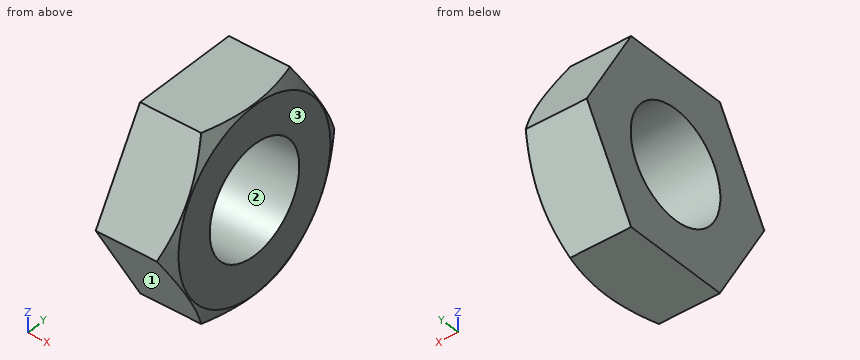
```python
from build123d import *

# Parameters (mm, degrees)
BOSS_EXTRUDE1_DEPTH        = 9
M16X2_0_TAPPED_HOLE1_D     = 14
M16X2_0_TAPPED_HOLE1_DEPTH = 9


with BuildPart() as part:
    # Sketch1 → Boss-Extrude1 (new body)
    with BuildSketch(Plane(origin=(0, 0, 0), x_dir=(0, 0, -1), z_dir=(1, 0, 0))):
        Polygon((12, 6.92820323), (0, 13.856406461), (-12, 6.92820323), (-12, -6.92820323), (0, -13.856406461), (12, -6.92820323), align=None)
    extrude(amount=-BOSS_EXTRUDE1_DEPTH)

    # M16x2.0 Tapped Hole1
    with Locations(Plane(origin=(0, 0, 0), x_dir=(0, 0, -1), z_dir=(1, 0, 0))):
        with Locations((0, 0)):
            Hole(M16X2_0_TAPPED_HOLE1_D / 2, depth=M16X2_0_TAPPED_HOLE1_DEPTH)

    # Sketch10 → Cut-Revolve1 (revolve, cut)
    with BuildSketch(Plane.XY):
        Polygon((0, 13.856406461), (0, 11.856406461), (-1.154700538, 13.856406461), align=None)
    revolve(axis=Axis((0, 0, 0), (1, 0, 0)), mode=Mode.SUBTRACT)


solid = part.part
```
Verification items for the finished model (mm, model axes). Face numbers are marked on the shaded views. Give positions to 0.01 mm unless a question says otherwise; leave off trailing zeros. Order: outer loops, then holes, each group sorted by start corner. A loop starts at its lowest first (then second) coordinate and runs counter-clockwise, first axis right, second up. Notation, with made-up numbers: (23.25, 74.5) -> (57.25, 74.5) arc R22 cw to (57.25, 102.5) -> close; hole circle Ø11 at (28, -5). An arc over 180 degrees is marked (long way). One line per item, written item: value.
(1) Draft check along Y on the marked faces 1, 2 and 3. Enter one of: pulls with the +Y half, pulls with the -Y half, needs draft (parallel to the pull), parting line crosses it, or undercut.
Final values:
face 1: pulls with the -Y half
face 2: undercut
face 3: needs draft
(2) Sectioned sample at A-A on x = -3.25. Record the cut outline in (y, z), then the cut area to 3 significant figures.
Final values:
outline: (-13.86, 0) -> (-6.93, -12) -> (6.93, -12) -> (13.86, 0) -> (6.93, 12) -> (-6.93, 12) -> close; hole circle Ø14 at (0, 0)
area: 345 mm^2
(3) Gauge pin test, flat ends, axial feed: pin 1 (1.5 mm diameter, centred on x = -7.5, y = 9, fed in from +Z); pin 2 (3 mm diameter, centred on x = -4.5, z = -9.5, fed in from +Y). Record the tip position at first contact, or that the pin passes through.
Final values:
pin 1: z = 9.71
pin 2: y = 9.24
(4) Sectioned sample at B-B on y = 0. Record the cut outline in (x, z), then the cut area to 3 significant figures.
Final values:
outline: (-9, -12) -> (-0.08, -12) -> (0, -11.86) -> (0, -7) -> (-9, -7) -> close; (-9, 7) -> (0, 7) -> (0, 11.86) -> (-0.08, 12) -> (-9, 12) -> close
area: 90.0 mm^2
(5) Scan lines: line 1 along Z through (x, y) = (-3.25, -1); line 2 along Z through (x, y) = (-4.75, 2.25); line 3 along Y through (x, z) = (-5, 0.25). Record each from-to range of solid material in increasing order. Write a range as [from, to].
Final values:
line 1: [-12, -6.93], [6.93, 12]
line 2: [-12, -6.63], [6.63, 12]
line 3: [-13.71, -7], [7, 13.71]
